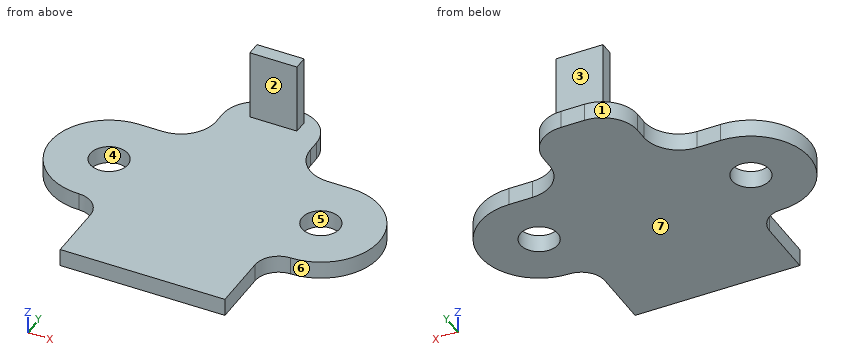
```python
from build123d import *

# Parameters (mm, degrees)
BOSS_EXTRUDE1_DEPTH        = 1.5
F_3_2_3_2_DIAMETER_HOLE1_D = 3.2
SKETCH5_W                  = 4
SKETCH5_H                  = 1.181538701
BOSS_EXTRUDE2_DEPTH        = 6


with BuildPart() as part:
    # Sketch1 → Boss-Extrude1 (new body)
    with BuildSketch(Plane.XY.offset(1.5)):
        with BuildLine():
            Line((-4, 9), (-4, 8))
            ThreePointArc((-4, 8), (-4.878679656, 5.878679656), (-7, 5))
            Line((-7, 5), (-9, 5))
            ThreePointArc((-9, 5), (-14, 0), (-9, -5))
            ThreePointArc((-9, -5), (-7.585786438, -5.585786438), (-7, -7))
            Line((-7, -7), (-7, -12))
            Line((-7, -12), (7, -12))
            Line((7, -12), (7, -7))
            ThreePointArc((7, -7), (7.585786438, -5.585786438), (9, -5))
            ThreePointArc((9, -5), (14, 0), (9, 5))
            Line((9, 5), (7, 5))
            ThreePointArc((7, 5), (4.878679656, 5.878679656), (4, 8))
            Line((4, 8), (4, 9))
            ThreePointArc((4, 9), (3.121320344, 11.121320344), (1, 12))
            Line((1, 12), (-1, 12))
            ThreePointArc((-1, 12), (-3.121320344, 11.121320344), (-4, 9))
        make_face()
    extrude(amount=-BOSS_EXTRUDE1_DEPTH)

    # Ø3.2 (3.2) Diameter Hole1 (through all)
    with Locations(Plane.XY.offset(1.5)):
        with Locations((-9, 0)):
            f_3_2_3_2_diameter_hole1 = Hole(F_3_2_3_2_DIAMETER_HOLE1_D / 2)

    # Mirror1: Ø3.2 (3.2) Diameter Hole1 across plane
    add(f_3_2_3_2_diameter_hole1.mirror(Plane(origin=(0, 0, 0), x_dir=(0, 0, 1), z_dir=(1, 0, 0))), mode=Mode.SUBTRACT)

    # Sketch5 → Boss-Extrude2 (add)
    with BuildSketch(Plane.XY.offset(1.5)):
        with Locations((0, 10.264616907)):
            Rectangle(SKETCH5_W, SKETCH5_H)
    extrude(amount=BOSS_EXTRUDE2_DEPTH)


solid = part.part
```
For this review, take the finished solid that the model builds, in its own axes (mm). Face numbers are marked on the shaded views. A direction names the side the tool comes from. Round coordinates to 2 decimals unless told otherwise and drop trailing zeros. Write each loop counter-clockwise with the first axis right and the second up, starting at its lowest first coordinate (ties: lowest second). Pieces come first, ordered by that corner, then holes. Notation, with made-up numbers: (-24.75, 45) - (23.25, 45) arc R30 ccw to (23.25, 83) - close; hole circle Ø5 at (67.5, 8). An arc over 180 degrees is marked (long way). Use CSV: the item, a comma, the result in double quotes.
1) Wall thickness on line 1 along Y through (x, z) = (9, 1.1); line 2 along Z through (x, y) = (-0.5, -7.75); line 3 along Y through (x, z) = (0.5, 2): over which ranges is each line inside the solid? List them lowest first. Write a range as from..to.
Conclusion:
line 1,"y = -5..-1.6, 1.6..5"
line 2,"z = 0..1.5"
line 3,"y = 9.67..10.86"
2) Add section B-B on z = 5.75. Write out the cut boundary in (x, y).
Conclusion:
outline,"(-2, 9.67) - (2, 9.67) - (2, 10.86) - (-2, 10.86) - close"
3) Clearance check with flat-ended pins moving along their axes: pin 1 Ø1.9 at (x, y) = (-9, 0) entering from +Z; pin 2 Ø0.8 at (x, z) = (7.5, 1) entering from +Y; pin 3 Ø0.6 at (y, z) = (10.5, 6) entering from +X; pin 4 Ø1.3 at (y, z) = (10, 5) entering from -X. State where each tip first meets the part, or that it passes through.
Conclusion:
pin 1,"passes through"
pin 2,"stops at y = 5"
pin 3,"stops at x = 2"
pin 4,"stops at x = -2"
4) The part is to be moulded in two halves that separate along X. For the marked faces 4, 5, 6 and 7, say which applies: pulls with the +X half, pulls with the -X half, needs draft (parallel to the pull), parting line crosses it, or undercut.
Conclusion:
face 4,"undercut"
face 5,"undercut"
face 6,"pulls with the +X half"
face 7,"needs draft"
5) Add section C-C on y = -3.75. Write out the cut boundary in (x, z).
Conclusion:
outline,"(-12.31, 0) - (12.31, 0) - (12.31, 1.5) - (-12.31, 1.5) - close"
6) Add section A-A on y = 0. Write out the cut boundary in (x, z).
Conclusion:
outline,"(-14, 0) - (-10.6, 0) - (-10.6, 1.5) - (-14, 1.5) - close; (-7.4, 0) - (7.4, 0) - (7.4, 1.5) - (-7.4, 1.5) - close; (10.6, 0) - (14, 0) - (14, 1.5) - (10.6, 1.5) - close"
7) For the marked faces 1, 2 and 3, list the 3-axis set-ups (+Z, -Z, +X, -X, +Y, -Y) from which the entire face can be reached by the end or side of a thin tool; tool diameter is ignored.
Conclusion:
face 1,"+Z, -Z, -X, +Y"
face 2,"+Z, +X, -X, -Y"
face 3,"+Z, +X, -X, +Y"
